Answer from the drawing. Dimensions are ordinates in mm from the lowest x, y and z of the part. A direction names the side the tool comes from. Round coordinates to 2 decimals unless told otherwise and drop trailing zeros. Write each loop counter-clockwise with the first axis right and the second up, starting at its lowest first coordinate (ties: lowest second). Pieces come first, ordered by that corner, then holes. Notation, with made-up numbers: (83, -6) -> (102, -6) arc R35 cw to (102, 28) -> close; hole circle Ø2 at (55.25, -18.75). An arc over 180 degrees is marked (long way). Answer as a JSON object with one key per item and string values. Group by question number.
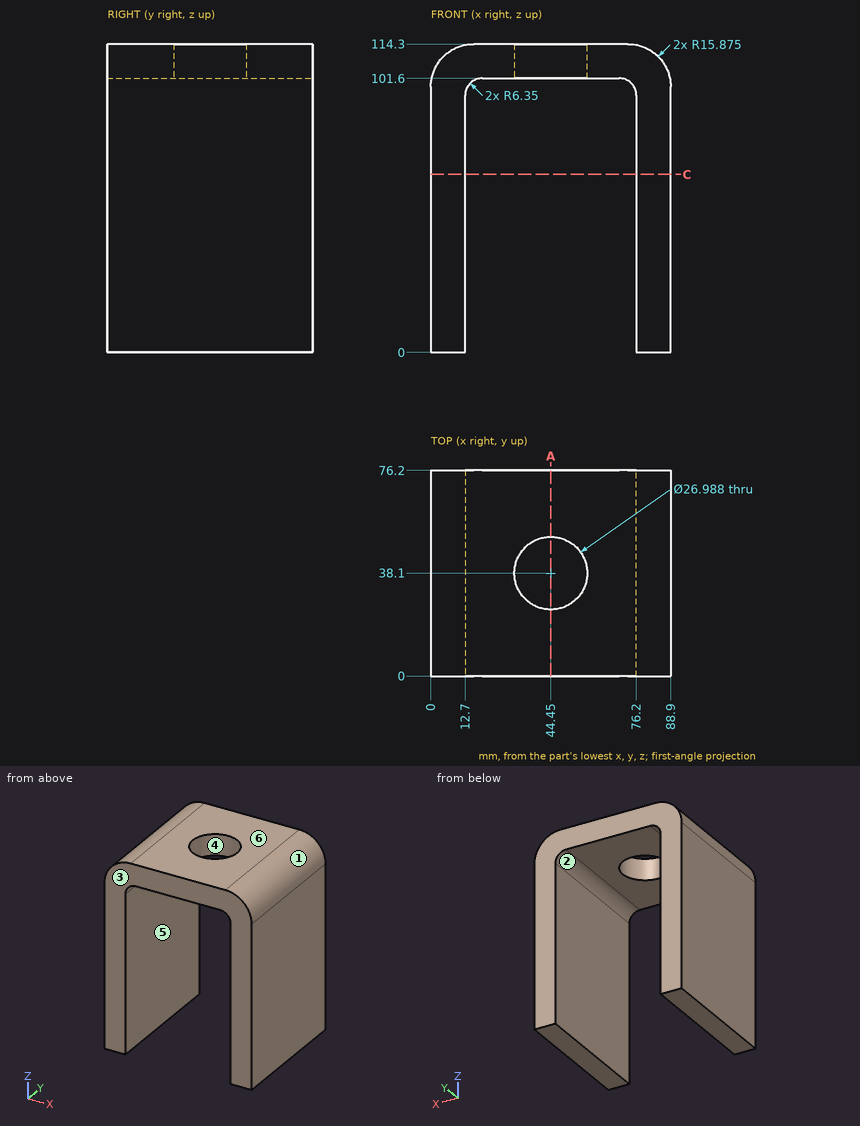
1) Each of these flat-tipped pins is pushed along its axis until it touches: P1, Ø1, axis at x = 54, y = 17, coming from the -Z side; P2, Ø21.5, axis at x = 44.45, y = 38.1, coming from the -Z side. Where does it stop, or does it pass through?
2) A cutting plane is placed at C-C on z = 66. Determine the outline of the cut face in (x, y).
3) A cutting plane is placed at A-A on x = 44.45. Determine the outline of the cut face in (y, z).
4) A tool of negligible diameter and unlimited length cuts with its end or side. For the marked faces 5 and 6, from which of +Z, -Z, +X, -X, +Y, -Y can it reach the whole face along a straight path? Write none if from no direction.
5) Straight lines are drawn through the part: L1, parallel to Y at x = 44.45, z = 106.25; L2, parallel to X at y = 35, z = 56.5; L3, parallel to Z at x = 69.5, y = 45. For each, find the intervals that lie inside material, in ascending order.
6) For a pull along X with two mould halves and no side action, classify the marked faces 1, 2, 3 and 4 as released by +X, released by -X, zero draft, split by the parting line, or undercut.
Established:
{
 "1": {"P1": "stops at z = 101.6", "P2": "passes through"},
 "2": {"outline": "(0, 0) -> (12.7, 0) -> (12.7, 76.2) -> (0, 76.2) -> close; (76.2, 0) -> (88.9, 0) -> (88.9, 76.2) -> (76.2, 76.2) -> close"},
 "3": {"outline": "(0, 101.6) -> (24.61, 101.6) -> (24.61, 114.3) -> (0, 114.3) -> close; (51.59, 101.6) -> (76.2, 101.6) -> (76.2, 114.3) -> (51.59, 114.3) -> close"},
 "4": {"face 5": "-Z, +Y, -Y", "face 6": "+Z, +X, -X, +Y, -Y"},
 "5": {"L1": "y = 0 to 24.61, 51.59 to 76.2", "L2": "x = 0 to 12.7, 76.2 to 88.9", "L3": "z = 101.6 to 114.3"},
 "6": {"face 1": "released by +X", "face 2": "undercut", "face 3": "zero draft", "face 4": "undercut"}
}
